Part model, mm, in its own coordinate system. Give positions to 0.01 mm unless a question says otherwise; leave off trailing zeros. Write each loop counter-clockwise with the first axis right and the second up, starting at its lowest first coordinate (ties: lowest second). Pieces come first, ordered by that corner, then holes. Notation, with made-up numbers: M 47,-36 L 63,-36 A24 cw 63,-4 Z; hole C 55,-36 d10. An arc over 180 degrees is marked long. Use a Markdown table: item, result. Add a question column.
from build123d import *

# Parameters (mm, degrees)
IZIM1_R                     = 0.75
IZIM1_R_2                   = 2.5
IZIM1_R_3                   = 2
Y_KSEKLIK_EKSTR_ZYON1_DEPTH = 2


with BuildPart() as part:
    # Çizim1 → Yükseklik-Ekstrüzyon1 (new body, symmetric)
    with BuildSketch(Plane.XY):
        with BuildLine():
            Line((-0.997183534, 20.075), (-2.492958834, 0.1875))
            ThreePointArc((-2.492958834, 0.1875), (0, 2.5), (2.492958834, 0.1875))
            Line((2.492958834, 0.1875), (0.997183534, 20.075))
            ThreePointArc((0.997183534, 20.075), (0, 21), (-0.997183534, 20.075))
        make_face()
        with Locations((0, 20)):
            Circle(IZIM1_R, mode=Mode.SUBTRACT)
        Circle(IZIM1_R_2)
        Circle(IZIM1_R_3, mode=Mode.SUBTRACT)
    extrude(amount=Y_KSEKLIK_EKSTR_ZYON1_DEPTH, both=True)


solid = part.part
1. Flat gauge pins, fed straight in: pin 1 (2 mm diameter, centred on y = 18.5, z = 1.5, fed in from -X); pin 2 (2 mm diameter, centred on x = 0, y = 20, fed in from +Z); pin 3 (1 mm diameter, centred on y = 5.5, z = 0.5, fed in from -X). Where does each tip first touch, or does it go through?
2. Cut at D-D (y = 19.75). Write the cut outline in (x, z).
3. Cut at C-C (x = 1.65). Write the cut outline in (y, z), then the cut area to 3 significant figures.
4. Cut at A-A (x = 0). Write the cut outline in (y, z), then the cut area to 3 significant figures.
5. Drill centre lines: probe 1 along Y at (x, z) = (0.2, 0.9); probe 2 along Y at (x, z) = (0.6, 0.95); probe 3 along Y at (x, z) = (0.8, -1.25). Where is each one in solid material? Low to high. Write a range as [from, to].
6. Mould opens along Y. For faces 1 (the flat face through (0, 9, -2)), 2 (the flat face through (1.756, 9.992, 0.028)), 3 (the cylindrical face through (-0.163, 19.268, -0.028)) say: released by +Y, released by -Y, zero draft, split by the parting line, or undercut.
7. Cut at B-B (z = -0.95). Give the number of separate pieces and of enclosed holes in the cut face, then the cut area to 3 significant figures.
A:
| question | item | result |
|---|---|---|
| 1 | pin 1 | stops at x = -1.19 |
| 1 | pin 2 | stops at z = 2 |
| 1 | pin 3 | stops at x = -2.13 |
| 2 | outline | M -1.02,-2 L -0.71,-2 L -0.71,2 L -1.02,2 Z; M 0.71,-2 L 1.02,-2 L 1.02,2 L 0.71,2 Z |
| 3 | outline | M -1.88,-2 L -1.13,-2 L -1.13,2 L -1.88,2 Z; M 1.13,-2 L 11.4,-2 L 11.4,2 L 1.13,2 Z |
| 3 | area | 44.1 mm² |
| 4 | outline | M -2.5,-2 L -2,-2 L -2,2 L -2.5,2 Z; M 2,-2 L 19.25,-2 L 19.25,2 L 2,2 Z; M 20.75,-2 L 21,-2 L 21,2 L 20.75,2 Z |
| 4 | area | 72.0 mm² |
| 5 | probe 1 | y = [-2.49, -1.99], [1.99, 19.28], [20.72, 20.98] |
| 5 | probe 2 | y = [-2.43, -1.91], [1.91, 19.55], [20.45, 20.8] |
| 5 | probe 3 | y = [-2.37, -1.83], [1.83, 20.6] |
| 6 | face 1 | zero draft |
| 6 | face 2 | released by +Y |
| 6 | face 3 | undercut |
| 7 | separate pieces | 1 |
| 7 | enclosed holes | 2 |
| 7 | area | 67.3 mm² |
